Study the drawing (mm; zero at the part's minimum x, y, z) and answer. A direction names the side the tool comes from. Round coordinates to 2 decimals unless told otherwise and drop trailing zeros. Write each loop counter-clockwise with the first axis right and the second up, starting at its lowest first coordinate (ties: lowest second). Pieces come first, ordered by that corner, then holes. Notation, with made-up numbers: (32.25, -1) - (76.25, -1) arc R23 cw to (76.25, 14) - close; hole circle Ø2 at (8, -26.5). An arc over 180 degrees is marked (long way). Return JSON: item names as keys, results as strings. Group by question number.
(1) Section C-C, the plane y = 31.3 is taken. Write down the section's boundary in (x, z).
(2) Section A-A, the plane z = 24 is taken. Write down the section's boundary in (x, y), then the cut area to 3 significant figures.
(3) Section B-B, the plane x = 18.5 is taken. Write down the section's boundary in (y, z), then the cut area to 3 significant figures.
(4) Find the intervals of material crossed by line 1 along Y through (x, z) = (21, 22.55); line 2 along X through (y, z) = (42, 21.2); line 3 along Y through (x, z) = (3.75, 24.5), in increasing order. Write a range as [from, to].
(5) Each of these flat-tipped pins is pushed along its axis until it touches: pin 1 (2 mm diameter, centred on y = 30, z = 27, fed in from +X); pin 2 (3 mm diameter, centred on x = 3, y = 3, fed in from -Z); pin 3 (1.2 mm diameter, centred on x = 2, z = 27.5, fed in from -Y); pin 4 (2 mm diameter, centred on x = 2, z = 26.5, fed in from +Y). Where does it stop, or does it pass through?
(6) Section D-D, the plane x = 22.75 is taken. Write down the section's boundary in (y, z), then the cut area to 3 significant figures.
(7) Determine the mould class of the marked faces 1, 2 and 3 for opening direction Y: +Y half, -Y half, draft (parallel to the pull), parting line (faces both ways), or undercut.
(8) Which of the six approach directions +Z, -Z, +X, -X, +Y, -Y give full straight-line access (tool end or side, diameter ignored) to the marked faces 4 and 5?
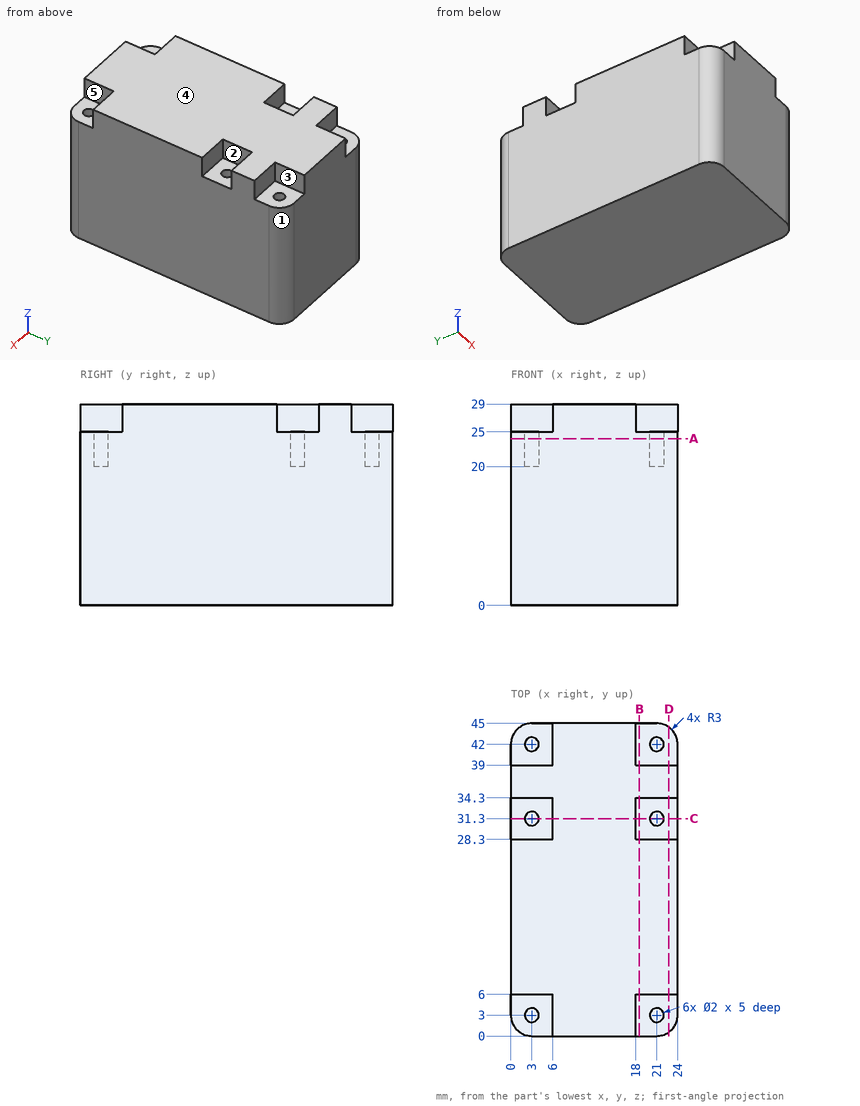
Working result:
{
 "1": {"outline": "(0, 0) - (24, 0) - (24, 25) - (22, 25) - (22, 20) - (20, 20) - (20, 25) - (18, 25) - (18, 29) - (6, 29) - (6, 25) - (4, 25) - (4, 20) - (2, 20) - (2, 25) - (0, 25) - close"},
 "2": {"outline": "(0, 3) arc R3 ccw to (3, 0) - (21, 0) arc R3 ccw to (24, 3) - (24, 42) arc R3 ccw to (21, 45) - (3, 45) arc R3 ccw to (0, 42) - close; hole circle Ø2 at (3, 3); hole circle Ø2 at (3, 31.3); hole circle Ø2 at (3, 42); hole circle Ø2 at (21, 3); hole circle Ø2 at (21, 31.3); hole circle Ø2 at (21, 42)", "area": "1,050 mm^2"},
 "3": {"outline": "(0, 0) - (45, 0) - (45, 25) - (39, 25) - (39, 29) - (34.3, 29) - (34.3, 25) - (28.3, 25) - (28.3, 29) - (6, 29) - (6, 25) - (0, 25) - close", "area": "1,230 mm^2"},
 "4": {"line 1": "y = [0, 2], [4, 30.3], [32.3, 41], [43, 45]", "line 2": "x = [0, 2], [4, 20], [22, 24]", "line 3": "y = [0, 2.34], [3.66, 30.64], [31.96, 41.34], [42.66, 45]"},
 "5": {"pin 1": "stops at x = 18", "pin 2": "stops at z = 0", "pin 3": "stops at y = 6", "pin 4": "stops at y = 39"},
 "6": {"outline": "(0.56, 0) - (44.44, 0) - (44.44, 25) - (39, 25) - (39, 29) - (34.3, 29) - (34.3, 25) - (28.3, 25) - (28.3, 29) - (6, 29) - (6, 25) - (0.56, 25) - close", "area": "1,200 mm^2"},
 "7": {"face 1": "+Y half", "face 2": "undercut", "face 3": "draft"},
 "8": {"face 4": "+Z, +X, -X, +Y, -Y", "face 5": "+Z, +X, -Y"}
}
